Verification items for the finished model (mm, model axes). Face numbers are marked on the shaded views. Coordinates: 2 decimals unless noted, no trailing zeros. Write each loop counter-clockwise with the first axis right and the second up, starting at its lowest first coordinate (ties: lowest second). Pieces come first, ordered by that corner, then holes. Notation, with made-up numbers: (88.5, 18.25) - (95.5, 18.25) arc R19 ccw to (95.5, 37.25) - close; hole circle Ø7 at (57.25, 2). An arc over 180 degrees is marked (long way). Use CSV: the item, a comma, the result in double quotes. Start each with the question number.
```python
from build123d import *

# Parameters (mm, degrees)
SKETCH1_R           = 1.705
BOSS_EXTRUDE1_DEPTH = 12


with BuildPart() as part:
    # Sketch1 → Boss-Extrude1 (new body)
    with BuildSketch(Plane.XY):
        Polygon((-3.397125795, 3.5), (-5.602874205, -3.5), (5.602874205, -3.5), (5.602874205, 3.5), align=None)
        with Locations((1.102874205, 0)):
            Circle(SKETCH1_R, mode=Mode.SUBTRACT)
    extrude(amount=BOSS_EXTRUDE1_DEPTH)


solid = part.part
```
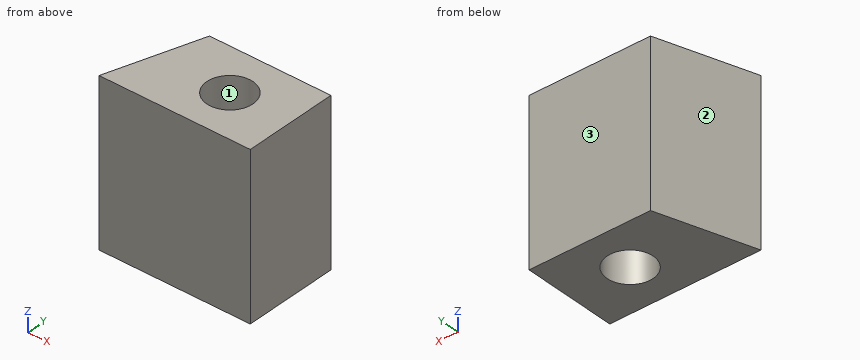
Q1. Cross-section at A-A (y = 0). Record the cut outline in (x, z), plus the area to 3 significant figures.
Q2. Gauge pin test, flat end, axial feed: pin 1 (3 mm diameter, centred on x = 3.5, y = 0, fed in from -Z). Record the tip position at first contact, or that the pin passes through.
Q3. Release check for a two-part mould opening along X. For the marked faces 1, 2 and 3 record: released by +X, released by -X, zero draft, split by the parting line, or undercut.
Q4. Cross-section at C-C (y = -1). Record the cut outline in (x, z), plus the area to 3 significant figures.
Q5. Cross-section at B-B (z = 1.5). Record the cut outline in (x, y) (3 decimals).
Q6. Scan lines: line 1 along X through (y, z) = (0.75, 2.25); line 2 along X through (y, z) = (-0.5, 1); line 3 along Y through (x, z) = (1.5, 2.75). Record each from-to range of solid material in increasing order. Write a range as from..to.
Q7. Cross-section at D-D (x = -4.5). Record the cut outline in (y, z), plus the area to 3 significant figures.
Reply:
1,outline,"(-4.5, 0) - (-0.6, 0) - (-0.6, 12) - (-4.5, 12) - close; (2.81, 0) - (5.6, 0) - (5.6, 12) - (2.81, 12) - close"
1,area,"80.3 mm^2"
2,pin 1,"z = 0"
3,face 1,"undercut"
3,face 2,"released by -X"
3,face 3,"zero draft"
4,outline,"(-4.82, 0) - (-0.28, 0) - (-0.28, 12) - (-4.82, 12) - close; (2.48, 0) - (5.6, 0) - (5.6, 12) - (2.48, 12) - close"
4,area,"91.9 mm^2"
5,outline,"(-5.603, -3.5) - (5.603, -3.5) - (5.603, 3.5) - (-3.397, 3.5) - close; hole circle Ø3.41 at (1.103, 0)"
6,line 1,"-4.26..-0.43, 2.63..5.6"
6,line 2,"-4.66..-0.53, 2.73..5.6"
6,line 3,"-3.5..-1.66, 1.66..3.5"
7,outline,"(-3.5, 0) - (0, 0) - (0, 12) - (-3.5, 12) - close"
7,area,"42.0 mm^2"
